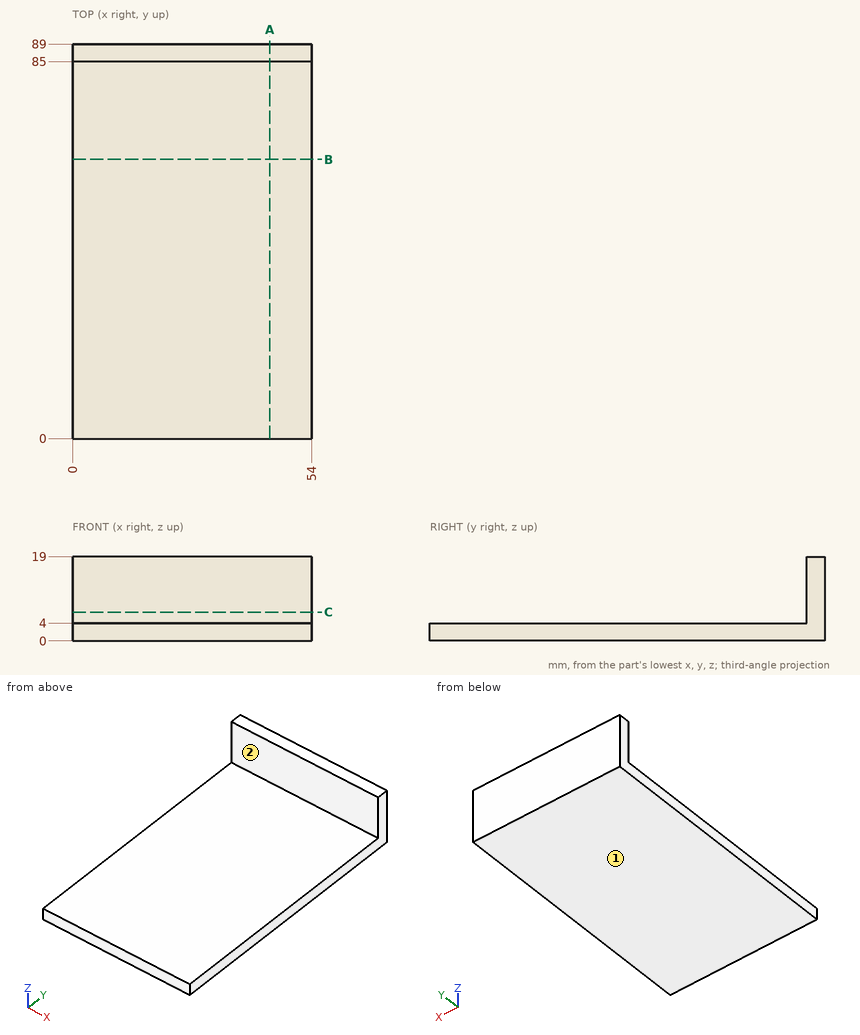
Answer from the drawing. Dimensions are ordinates in mm from the lowest x, y and z of the part. A direction names the side the tool comes from. Give positions to 0.01 mm unless a question says otherwise; leave off trailing zeros. Loops run counter-clockwise (first coordinate to the right, second up) from the corner with the lowest first, then second, coordinate; pieces in that order, holes last.
Item 1: A cutting plane is placed at A-A (x = 44.5). Give the vertices of the cut face in (y, z), then the cut area to 3 significant figures.
Derived:
outline: (0, 0) - (89, 0) - (89, 19) - (85, 19) - (85, 4) - (0, 4) - close
area: 416 mm2
Item 2: A cutting plane is placed at B-B (y = 63). Give the vertices of the cut face in (x, z), then the cut area to 3 significant figures.
Derived:
outline: (0, 0) - (54, 0) - (54, 4) - (0, 4) - close
area: 216 mm2
Item 3: A tool of negligible diameter and unlimited length cuts with its end or side. For the marked faces 1 and 2, from which of +Z, -Z, +X, -X, +Y, -Y can it reach the whole face along a straight path? Write none if from no direction.
Derived:
face 1: -Z, +X, -X, +Y, -Y
face 2: +Z, +X, -X, -Y
Item 4: Each of these flat-tipped pins is pushed along its axis until it touches: pin 1 Ø2 at (x, y) = (27, 20) entering from +Z; pin 2 Ø5 at (y, z) = (55, 8) entering from -X; pin 3 Ø4.5 at (x, z) = (36.5, 11) entering from -Y. Where does it stop, or does it pass through?
Derived:
pin 1: stops at z = 4
pin 2: passes through
pin 3: stops at y = 85
Item 5: A cutting plane is placed at C-C (z = 6.5). Give the vertices of the cut face in (x, y), then the cut area to 3 significant figures.
Derived:
outline: (0, 85) - (54, 85) - (54, 89) - (0, 89) - close
area: 216 mm2
Item 6: Find the intervals of material crossed by line 1 along Z through (x, y) = (5, 44); line 2 along Y through (x, z) = (7.5, 8.5), in increasing order.
Derived:
line 1: z = 0 to 4
line 2: y = 85 to 89
